from build123d import *

# Parameters (mm, degrees)
F0_R     = 2.5
F1_DEPTH = 5
F2_R     = 4.99999


# Not quite as in the source:
# - a fillet or chamfer is up to 0.001 mm smaller than in the source, because OpenCascade refuses the exact size


with BuildPart() as f1:
    # F0 (on Top) → F1 (new body)
    with BuildSketch(Plane.XY):
        Polygon((0, 50), (0, 0), (10, 0), (10, 100), (0, 100), align=None)
        with Locations((5, 50)):
            Circle(F0_R, mode=Mode.SUBTRACT)
        with Locations((5, 90)):
            Circle(F0_R, mode=Mode.SUBTRACT)
    extrude(amount=F1_DEPTH)

    # F2 (radius 5 in the source; OpenCascade refuses exactly that, so slightly less here)
    f2_edges = [f1.edges().sort_by_distance(p)[0] for p in [
        (0, 100, 2.5),
        (10, 100, 2.5),
    ]]
    fillet(f2_edges, radius=F2_R)


solid = f1.part
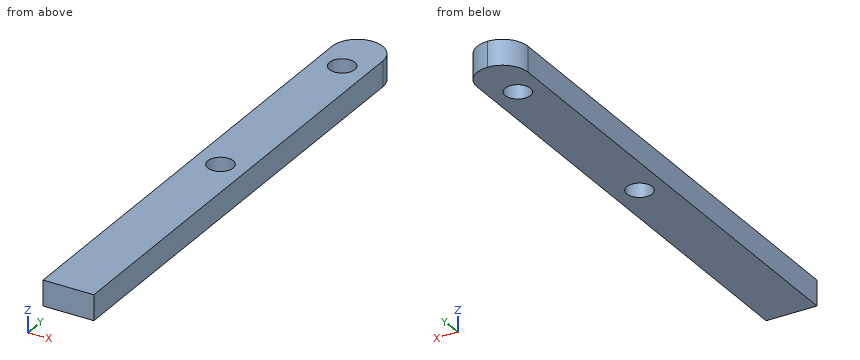
The model under review builds one solid part; all positions refer to its coordinate system, in mm. Round coordinates to 2 decimals unless told otherwise and drop trailing zeros. Loops run counter-clockwise (first coordinate to the right, second up) from the corner with the lowest first, then second, coordinate; pieces in that order, holes last. Notation, with made-up numbers: M 89.25,-25 L 96.25,-25 A18 cw 96.25,10 Z; hole C 19.5,23.25 d6. An arc over 180 degrees is marked long. Answer as CSV lines item,"result". Start each with the question number.
Item 1: Consider section A-A (y = 90). Write out the cut boundary in (x, z).
Item 2: Wall thickness on line 1 (Y direction, x = 5, z = 2); line 2 (Y direction, x = 1, z = 4.1); line 3 (Y direction, x = 7.75, z = 3.8): over which ranges is each line inside the solid? List them lowest first. Write a range as [from, to].
Item 3: Consider section C-C (x = 8.75). Write out the cut boundary in (y, z).
Item 4: Insertion check: P1, Ø3, axis at x = 6.5, z = 1.5, coming from the -Y side. The pin has a flat end and moves straight along its axis. Give the tip position at first contact, or say it passes through.
Item 5: Consider section B-B (z = 2.6). State how many separate pieces and enclosed holes the cut face has, then the cut area to 3 significant figures.
Answer:
1,outline,"M 0,0 L 2.5,0 L 2.5,5 L 0,5 Z; M 7.5,0 L 10,0 L 10,5 L 7.5,5 Z"
2,line 1,"y = [0, 47.5], [52.5, 87.5], [92.5, 100]"
2,line 2,"y = [0, 98]"
2,line 3,"y = [0, 99.18]"
3,outline,"M 0,0 L 98.31,0 L 98.31,5 L 0,5 Z"
4,P1,"stops at y = 0"
5,separate pieces,"1"
5,enclosed holes,"2"
5,area,"950 mm^2"
